The listing builds one solid part. Answer for the finished solid, in the listing's coordinates (mm). A direction names the side the tool comes from. Give positions to 0.01 mm unless a question says otherwise; leave off trailing zeros. Order: outer loops, then holes, each group sorted by start corner. A loop starts at its lowest first (then second) coordinate and runs counter-clockwise, first axis right, second up. Notation, with made-up numbers: (24.5, 18) - (81.5, 18) arc R9 cw to (81.5, 28) - close; hole circle Ø8 at (7.25, 3). An arc over 180 degrees is marked (long way). Use CSV: the item, a comma, the result in double quotes.
Autodesk Inventor part; units mm, degrees
ref_plane "YZ Plane" through (0, 0, 0) normal (1, 0, 0) x (0, 1, 0)
ref_plane "XZ Plane" through (0, 0, 0) normal (0, 1, 0) x (-1, 0, 0)
ref_plane "XY Plane" through (0, 0, 0) normal (0, 0, 1) x (1, 0, 0)
sketch "Sketch3" plane through (0, 0, 0) normal (0, 0, 1) x (1, 0, 0)
  line L0 (-48.8137, 10.438) -> (-52.9368, 29.0364) construction
  line L1 (-52.9368, 29.0364) -> (-59.1363, 27.662) construction
  line L2 (-59.1363, 27.662) -> (-55.0132, 9.0636) construction
  line L3 (-55.0132, 9.0636) -> (-48.8137, 10.438) construction
  line L4 (-48.8137, 10.438) -> (-59.1363, 27.662) construction
  line L5 (-52.9368, 29.0364) -> (-55.0132, 9.0636) construction
  circle A0 centre (-50.8753, 19.7372) radius 1.7526
  circle A1 centre (-59.1363, 27.662) radius 1.7526
  circle A2 centre (-55.0132, 9.0636) radius 1.7526
  line L6 (0, 0) -> (-127, 0)
  line L7 (0, 60.0769) -> (0, 0) construction
  line L8 (-44.6831, 6.4756) -> (-50.8679, 34.3732)
  line L9 (-50.8679, 34.3732) -> (-63.2669, 31.6244) construction
  line L10 (-63.2669, 31.6244) -> (-57.0821, 3.7268) construction
  line L11 (-57.0821, 3.7268) -> (-44.6831, 6.4756) construction
  line L12 (-44.6831, 6.4756) -> (-63.2669, 31.6244) construction
  line L13 (-50.8679, 34.3732) -> (-57.0821, 3.7268) construction
  line L14 (-45.2216, 8.9044) -> (-50.032, 30.6026)
  line L15 (-50.8679, 34.3732) -> (0, 45.6504) construction
  arc A3 (-128.0308, 9.4121) -> (-127, 0) centre (-127, 4.7625) ccw
  line L16 (-127, 0) -> (-127, 4.7625) construction
  line L17 (-128.0308, 9.4121) -> (-65.3965, 23.2978)
  line L18 (-9.6463, 43.5118) -> (0, 0)
  circle A4 centre (-127, 4.7625) radius 1.7526
  line L19 (-111.125, 0) -> (-12.7, 0) construction
  line L20 (-12.7, 0) -> (-12.7, 4.7625) construction
  line L21 (-12.7, 4.7625) -> (-111.125, 4.7625) construction
  line L22 (-111.125, 4.7625) -> (-111.125, 0) construction
  line L23 (-12.7, 2.3812) -> (-111.125, 2.3812) construction
  circle A5 centre (-108.7437, 2.3812) radius 1.4732
  circle A6 centre (-96.0437, 2.3812) radius 1.4732
  circle A7 centre (-83.3438, 2.3812) radius 1.4732
  circle A8 centre (-70.6437, 2.3812) radius 1.4732
  circle A9 centre (-57.9438, 2.3812) radius 1.4732
  circle A10 centre (-45.2438, 2.3812) radius 1.4732
  circle A11 centre (-32.5438, 2.3812) radius 1.4732
  circle A12 centre (-19.8438, 2.3812) radius 1.4732
  circle A13 centre (-8.5171, 19.3715) radius 1.7526
  line L24 (-55.0132, 9.0636) -> (-8.5171, 19.3715) construction
  line L25 (-53.9824, 4.414) -> (-8.0676, 14.593) construction
  line L26 (-5.5232, 24.9134) -> (-56.0439, 13.7132)
  arc A14 (-56.0439, 13.7132) -> (-53.9824, 4.414) centre (-55.0132, 9.0636) ccw construction
  line L27 (-5.5232, 24.9134) -> (-76.0422, 9.2797)
  line L28 (-76.0422, 9.2797) -> (-78.5057, 20.3916)
  line L29 (-78.5057, 20.3916) -> (-7.9866, 36.0253)
  line L30 (-7.9866, 36.0253) -> (-5.5232, 24.9134)
  line L31 (-50.5317, 18.1873) -> (-129.4495, 8.8468)
  line L32 (-59.1437, 13.026) -> (-76.0422, 13.026) construction
  line L33 (-76.0422, 13.026) -> (-76.0422, 6.35) construction
  line L34 (-76.0422, 6.35) -> (-59.1437, 6.35)
  line L35 (-59.1437, 6.35) -> (-59.1437, 13.026)
  arc A15 (-76.0422, 9.2797) -> (-72.3919, 6.35) centre (-72.3919, 10.0889) ccw
  line L36 (-127, 0) -> (-136.525, 0)
  line L37 (-136.525, 0) -> (-136.525, 12.7)
  line L38 (-136.525, 12.7) -> (-127, 12.7)
  line L39 (-127, 12.7) -> (-127, 0)
  arc A16 (-133.7857, 12.7) -> (-129.4495, 8.8468) centre (-129.9056, 12.7) ccw
  circle A17 centre (-8.5171, 19.3715) radius 4.1224
  line L40 (-12.7, 0) -> (-4.7567, 17.6823)
  point P0 (-53.975, 19.05)
  point P1 (-53.975, 19.05)
  point P2 (-53.975, 19.05)
  point P3 (-127, 0)
  point P4 (-46.7447, 15.7748)
  point P5 (-78.5057, 20.3916)
  point P6 (-77.3143, 15.0174)
  point P7 (-4.4924, 20.2638)
  dimension "d71" = 19.05
  dimension "d72" = 6.35
  dimension "d73" = 3.5052
  dimension "d74" = 3.5052
  dimension "d75" = 3.5052
  dimension "d76" = 127
  dimension "d77" = 19.05
  dimension "d78" = 12.5
  dimension "d91" = 12.7
  dimension "d92" = 28.575
  dimension "d93" = 53.975
  dimension "d98" = 9.525
  dimension "d107" = 3.5052
  dimension "d108" = 98.425
  dimension "d109" = 4.7625
  dimension "d110" = 15.875
  dimension "d111" = 2.9464
  dimension "d112" = 2.3813
  dimension "d115" = 12.7
  dimension "d120" = 3.5052
  dimension "d127" = 3.175
  dimension "d129" = 6.75
  dimension "d135" = 47.625
  dimension "d136" = 72.2313
  dimension "d137" = 4.7625
  dimension "d138" = 6.35
  dimension "d139" = 9.525
  dimension "d140" = 12.7
extrude "Extrusion3" add sketch "Sketch3" along normal blind 6.35 contours L28 A15 L34 L35 L27 L26 L18 A17 L40 L6 L39 A4 L31 | L39 A4 A3 L31 | A3 L36 L37 L38 A16 | A17
extrude "Extrusion4" cut sketch "Sketch3" along normal through all contours A13
fillet "Fillet7" radius 3.175 2 edges at (-59.1437, 13.026, 3.175) (-59.1437, 6.35, 3.175)
equation "\"Angle_Mount\" = 105deg"
equation "\"Rail_Offset\" = 36.5125"
properties part number "Uprights" material "UHMW, White"
Item 1: Each of these flat-tipped pins is pushed along its axis until it touches: pin 1 (3 mm diameter, centred on y = 13, z = 5, fed in from +X); pin 2 (3 mm diameter, centred on x = -135, z = 2.5, fed in from +Y); pin 3 (1 mm diameter, centred on x = -90.5, z = 4, fed in from +Y). Where does it stop, or does it pass through?
Taken from the geometry:
pin 1,"x = -6.19"
pin 2,"y = 12.7"
pin 3,"y = 13.52"
Item 2: The mould has two halves that part along Y. Classify faces 4 (the face through (-60.098, 7.255, 3.219)), 5 (the face through (-4.414, 18.97, 3.131)), 6 (the face through (-53.394, 9.735, 3.131)): +Y half, -Y half, draft (parallel to the pull), parting line (faces both ways), or undercut.
Taken from the geometry:
face 4,"+Y half"
face 5,"parting line"
face 6,"undercut"
Item 3: Find the intervals of material crossed by line 1 along X through (y, z) = (8.25, 4) (1 decimal); line 2 along X through (y, z) = (8.5, 0.5) (3 decimals); line 3 along Y through (x, z) = (-64.5, 2.5), in increasing order.
Taken from the geometry:
line 1,"-136.5 to -75.6, -59.4 to -56.6, -53.5 to -9"
line 2,"-136.525 to -75.776, -59.314 to -56.673, -53.354 to -8.882"
line 3,"0 to 6.35"
Item 4: The part is cut by section B-B (z = 3.5). Count the separate pieces of the cut face and the enclosed holes in it, and give its area (3 significant figures).
Taken from the geometry:
separate pieces,"1"
enclosed holes,"11"
area,"1,710 mm^2"
Item 5: The part is cut by section C-C (x = -27). Give the vertices of the cut face in (y, z), and give its area (3 significant figures).
Taken from the geometry:
outline,"(0, 0) - (20.15, 0) - (20.15, 6.35) - (0, 6.35) - close"
area,"128 mm^2"
Item 6: Which of the six approach directions +Z, -Z, +X, -X, +Y, -Y give full straight-line access (tool end or side, diameter ignored) to faces 1 (the face through (-46.716, 2.316, 3.131)), 2 (the face through (-135, 12.7, 3)), 3 (the face through (-58.426, 12.488, 3.219))?
Taken from the geometry:
face 1,"+Z, -Z"
face 2,"+Z, -Z, -X, +Y"
face 3,"+Z, -Z, +Y"
Item 7: The part is cut by section A-A (x = -127). Give the vertices of the cut face in (y, z).
Taken from the geometry:
outline,"(0, 0) - (3.01, 0) - (3.01, 6.35) - (0, 6.35) - close; (6.52, 0) - (9.14, 0) - (9.14, 6.35) - (6.52, 6.35) - close"
